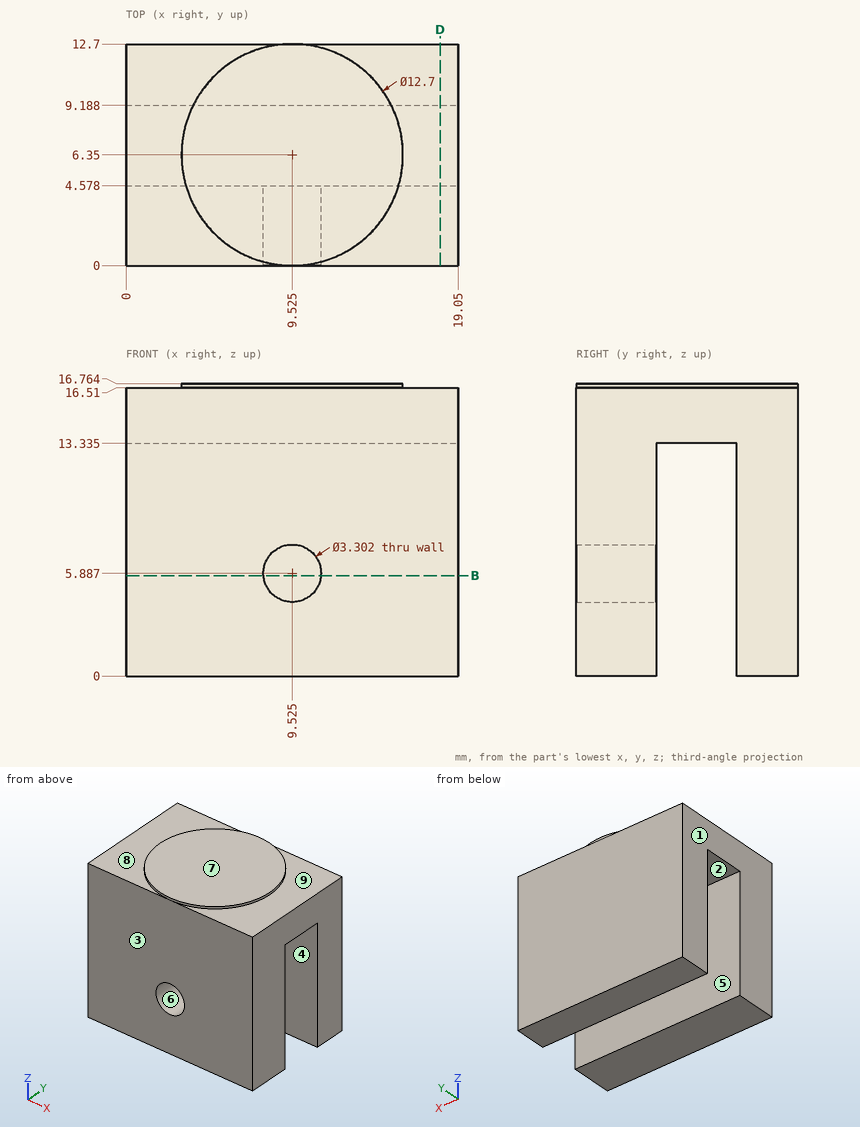
Input: dimensioned drawing with shaded views. Units: mm. Origin: part minimum x, y, z. A direction names the side the tool comes from. Give positions to 0.01 mm unless a question says otherwise; leave off trailing zeros. Loops run counter-clockwise (first coordinate to the right, second up) from the corner with the lowest first, then second, coordinate; pieces in that order, holes last. Notation, with made-up numbers: M 17.25,-11 L 45.25,-11 A38 cw 45.25,28 Z; hole C -34.5,-33.5 d4. An arc over 180 degrees is marked long. Put each result on its own line as item: value. Start each with the question number.
1) Cut plane D-D (x = 18). Output: boundary loops of the cut face in (y, z) (1 decimal).
2) Cut plane B-B (z = 5.75). Output: boundary loops of the cut face in (x, y).
3) Contact query for flat-ended pins moving along their axis: pin 1 (2 mm diameter, centred on y = 8, z = 11.5, fed in from +X); pin 2 (1 mm diameter, centred on x = 12.5, y = 6.5, fed in from -Z) (3 decimals); pin 3 (4 mm diameter, centred on x = 8.5, z = 5.5, fed in from -Y). Output: stop coordinate, or through.
4) Access query for the marked faces 5, 6, 7, 8 and 9. Directions: +Z, -Z, +X, -X, +Y, -Y. A direction counts if a zero-diameter tool reaches every point of the face in a straight line with its end or side. Return the directions, or none.
5) Pull-direction query (Y, two-part tool) for the marked faces 1, 2, 3 and 4; classes: pulls with the +Y half, pulls with the -Y half, needs draft (parallel to the pull), parting line crosses it, or undercut.
6) Ray query, line 1 along Y through (x, z) = (12.5, 11.5); line 2 along Z through (x, y) = (17.5, 10.25); line 3 along Z through (x, y) = (8.75, 7.5) (1 decimal). Return the intervals inside material, ascending.
Verdict:
1. outline: M 0,0 L 4.6,0 L 4.6,13.3 L 9.2,13.3 L 9.2,0 L 12.7,0 L 12.7,16.5 L 0,16.5 Z
2. outline: M 0,0 L 7.88,0 L 7.88,4.58 L 0,4.58 Z; M 0,9.19 L 19.05,9.19 L 19.05,12.7 L 0,12.7 Z; M 11.17,0 L 19.05,0 L 19.05,4.58 L 11.17,4.58 Z
3. pin 1: through
3. pin 2: z = 13.335
3. pin 3: y = 0
4. face 5: -Z, +X, -X
4. face 6: -Y
4. face 7: +Z, +X, -X, +Y, -Y
4. face 8: +Z, -X
4. face 9: +Z, +X
5. face 1: needs draft
5. face 2: undercut
5. face 3: pulls with the -Y half
5. face 4: undercut
6. line 1: 0 to 4.58, 9.19 to 12.7
6. line 2: 0 to 16.51
6. line 3: 13.3 to 16.8
